from build123d import *

# Parameters (mm, degrees)
SKETCH_1_W          = 110
SKETCH_1_H          = 55
SKETCH_1_R          = 1.7
EXTRUDE_1_DEPTH     = 3
SKETCH_2_W          = 103.5
SKETCH_2_H          = 38
EXTRUDE_2_DEPTH     = 3
SKETCH_3_R          = 1.6
CUT_EXTRUDE_1_DEPTH = 4
SKETCH_4_W          = 80
SKETCH_4_H          = 50
SKETCH_4_W_2        = 66.999999997
SKETCH_4_H_2        = 13.999999819
CUT_EXTRUDE_2_DEPTH = 4
FILLET_2_R          = 10
FILLET_3_R          = 1
FILLET_5_R          = 5
SKETCH_10_R         = 1.65
CUT_EXTRUDE_5_DEPTH = 4
SKETCH_11_W         = 55
SKETCH_11_H         = 9
CUT_EXTRUDE_6_DEPTH = 4
FILLET_6_R          = 2


with BuildPart() as part:
    # 草图1 → 凸台-拉伸1 (new body)
    with BuildSketch(Plane.XY):
        Rectangle(SKETCH_1_W, SKETCH_1_H)
        with Locations((-47.5, 12.5)):
            Circle(SKETCH_1_R, mode=Mode.SUBTRACT)
        with Locations((-47.5, -12.5)):
            Circle(SKETCH_1_R, mode=Mode.SUBTRACT)
        with Locations((47.5, 12.5)):
            Circle(SKETCH_1_R, mode=Mode.SUBTRACT)
        with Locations((47.5, -12.5)):
            Circle(SKETCH_1_R, mode=Mode.SUBTRACT)
    extrude(amount=EXTRUDE_1_DEPTH)

    # 草图2 → 凸台-拉伸2 (add)
    with BuildSketch(Plane.XY.offset(3)):
        with Locations((0, 46.5)):
            Rectangle(SKETCH_2_W, SKETCH_2_H)
    extrude(amount=-EXTRUDE_2_DEPTH)

    # 草图3 → 切除-拉伸1 (cut, through all)
    with BuildSketch(Plane(origin=(0, 0, 0), x_dir=(-1, 0, 0), z_dir=(0, 0, -1))):
        with Locations((37.35, 60.5)):
            Circle(SKETCH_3_R)
        with Locations((-37.649999997, 60.5)):
            Circle(SKETCH_3_R)
        with Locations((-37.649999997, 38.500000181)):
            Circle(SKETCH_3_R)
        with Locations((37.35, 38.500000181)):
            Circle(SKETCH_3_R)
    extrude(amount=-CUT_EXTRUDE_1_DEPTH, mode=Mode.SUBTRACT)

    # 草图4 → 切除-拉伸2 (cut, through all)
    with BuildSketch(Plane.XY.offset(3)):
        with Locations((0, -2.5)):
            Rectangle(SKETCH_4_W, SKETCH_4_H)
        with Locations((0.149999999, 49.500000091)):
            Rectangle(SKETCH_4_W_2, SKETCH_4_H_2)
    extrude(amount=-CUT_EXTRUDE_2_DEPTH, mode=Mode.SUBTRACT)

    # 圆角2
    fillet_2_edges = [part.edges().sort_by_distance(p)[0] for p in [
        (-40, 22.5, 1.5),
        (40, 22.5, 1.5),
    ]]
    fillet(fillet_2_edges, radius=FILLET_2_R)

    # 圆角3
    fillet_3_edges = [part.edges().sort_by_distance(p)[0] for p in [
        (51.75, 27.5, 1.5),
        (-51.75, 27.5, 1.5),
        (-55, 27.5, 1.5),
        (55, 27.5, 1.5),
    ]]
    fillet(fillet_3_edges, radius=FILLET_3_R)

    # 圆角5
    fillet_5_edges = [part.edges().sort_by_distance(p)[0] for p in [
        (-51.75, 65.5, 1.5),
        (51.75, 65.5, 1.5),
        (-33.35, 56.5, 1.5),
        (33.649999997, 56.5, 1.5),
        (33.649999997, 42.500000181, 1.5),
        (-33.35, 42.500000181, 1.5),
    ]]
    fillet(fillet_5_edges, radius=FILLET_5_R)

    # 草图10 → 切除-拉伸5 (cut, through all)
    with BuildSketch(Plane.XY.offset(3)):
        with Locations((-22.85, 60.5)):
            Circle(SKETCH_10_R)
        with Locations((5.15, 60.5)):
            Circle(SKETCH_10_R)
    extrude(amount=-CUT_EXTRUDE_5_DEPTH, mode=Mode.SUBTRACT)

    # 草图11 → 切除-拉伸6 (cut, through all)
    with BuildSketch(Plane.XY.offset(3)):
        with Locations((0.75, 61)):
            Rectangle(SKETCH_11_W, SKETCH_11_H)
    extrude(amount=-CUT_EXTRUDE_6_DEPTH, mode=Mode.SUBTRACT)

    # 圆角6
    fillet_6_edges = [part.edges().sort_by_distance(p)[0] for p in [
        (28.25, 56.5, 1.5),
        (28.25, 65.5, 1.5),
        (-26.75, 56.5, 1.5),
        (-26.75, 65.5, 1.5),
    ]]
    fillet(fillet_6_edges, radius=FILLET_6_R)


solid = part.part
Verification items for the finished model (mm, model axes). A direction names the side the tool comes from. Coordinates: 2 decimals unless noted, no trailing zeros. Order: outer loops, then holes, each group sorted by start corner. A loop starts at its lowest first (then second) coordinate and runs counter-clockwise, first axis right, second up. Notation, with made-up numbers: (76, -19.5) -> (101, -19.5) arc R22 cw to (101, -12.5) -> close; hole circle Ø5 at (43, 15.25). An arc over 180 degrees is marked (long way). Put each result on its own line as item: value. Start each with the question number.
1. Mould release check, pull along X, two halves, no side actions. Record for faces 4 (the flat face through (55, -1, 1)), 5 (the cylindrical face through (45.8, 12.57, 1.48)), 6 (the flat face through (-1, 30, 0)), 7 (the flat face through (-33.35, 49, 2)): released by +X, released by -X, zero draft, split by the parting line, or undercut.
2. Material ranges on L1, parallel to Y at x = -47.5, z = 2.2; L2, parallel to X at y = 6.5, z = 1.65; L3, parallel to X at y = 39, z = 1.45, recorded low to high. Write a range as [from, to].
3. Cross-section at B-B, the plane x = -37.35. Record the boundary of the cut face in (y, z), then the cut area to 3 significant figures.
4. Cross-section at C-C, the plane y = 50. Record the boundary of the cut face in (x, z), then the cut area to 4 significant figures.
5. Cross-section at A-A, the plane y = -12.5. Record the boundary of the cut face in (x, z).
6. Go/stop test with flat-tipped pins: pin 1 Ø0.9 at (y, z) = (62, 1.5) entering from +X; pin 2 Ø1.5 at (y, z) = (50, 1) entering from +X; pin 3 Ø1 at (x, z) = (53, 1) entering from +Y. Record where each tip stops, or that it passes through.
7. Access from +Z, -Z, +X, -X, +Y, -Y to the whole of each face (thin tool, end or side, straight path). Record for faces 1 (the flat face through (-40, -8, 2)), 2 (the flat face through (33.65, 49, 2)), 3 (the flat face through (-26.75, 61, 2)).
8. Cross-section at D-D, the plane y = 38.5. Record the boundary of the cut face in (x, z).
Computed:
1. face 4: released by +X
1. face 5: undercut
1. face 6: zero draft
1. face 7: undercut
2. L1: [-27.5, -14.2], [-10.8, 10.8], [14.2, 65.44]
2. L2: [-55, -40], [40, 55]
2. L3: [-51.75, -38.87], [-35.83, 36.13], [39.17, 51.75]
3. outline: (19.28, 0) -> (36.9, 0) -> (36.9, 3) -> (19.28, 3) -> close; (40.1, 0) -> (58.9, 0) -> (58.9, 3) -> (40.1, 3) -> close; (62.1, 0) -> (65.5, 0) -> (65.5, 3) -> (62.1, 3) -> close
3. area: 119 mm2
4. outline: (-51.75, 0) -> (-33.35, 0) -> (-33.35, 3) -> (-51.75, 3) -> close; (33.65, 0) -> (51.75, 0) -> (51.75, 3) -> (33.65, 3) -> close
4. area: 109.5 mm2
5. outline: (-55, 0) -> (-49.2, 0) -> (-49.2, 3) -> (-55, 3) -> close; (-45.8, 0) -> (-40, 0) -> (-40, 3) -> (-45.8, 3) -> close; (40, 0) -> (45.8, 0) -> (45.8, 3) -> (40, 3) -> close; (49.2, 0) -> (55, 0) -> (55, 3) -> (49.2, 3) -> close
6. pin 1: x = 51.64
6. pin 2: x = 51.75
6. pin 3: y = 27.53
7. face 1: +Z, -Z, -Y
7. face 2: +Z, -Z
7. face 3: +Z, -Z, +Y
8. outline: (-51.75, 0) -> (-38.95, 0) -> (-38.95, 3) -> (-51.75, 3) -> close; (-35.75, 0) -> (36.05, 0) -> (36.05, 3) -> (-35.75, 3) -> close; (39.25, 0) -> (51.75, 0) -> (51.75, 3) -> (39.25, 3) -> close
